from build123d import *

# Parameters (mm, degrees)
SKETCH1_R           = 11
SKETCH1_R_2         = 9.5
BOSS_EXTRUDE1_DEPTH = 10
BOSS_EXTRUDE2_START = -3
SKETCH2_R           = 11
SKETCH2_R_2         = 10
BOSS_EXTRUDE2_DEPTH = 3
SKETCH4_R           = 9.5
SKETCH4_R_2         = 8.5
BOSS_EXTRUDE3_DEPTH = 4


with BuildPart() as part:
    # Sketch1 → Boss-Extrude1 (new body)
    with BuildSketch(Plane.XY):
        with BuildLine():
            Line((-27.5, -15), (27.5, -15))
            ThreePointArc((27.5, -15), (42.5, 0), (27.5, 15))
            Line((27.5, 15), (9.069178574, 15))
            ThreePointArc((9.069178574, 15), (0, 18.5), (-9.069178574, 15))
            Line((-9.069178574, 15), (-27.5, 15))
            ThreePointArc((-27.5, 15), (-42.5, 0), (-27.5, -15))
        make_face()
        with Locations((-27.5, 0)):
            Circle(SKETCH1_R, mode=Mode.SUBTRACT)
        with Locations((27.5, 0)):
            Circle(SKETCH1_R, mode=Mode.SUBTRACT)
        with Locations((0, 5)):
            Circle(SKETCH1_R_2, mode=Mode.SUBTRACT)
    extrude(amount=BOSS_EXTRUDE1_DEPTH)

    # Sketch2 → Boss-Extrude2 (add)
    # profile 1 of 2: a face of its own
    with BuildSketch(Plane.XY.offset(10).offset(BOSS_EXTRUDE2_START)):
        with Locations((-27.5, 0)):
            Circle(SKETCH2_R)
        with Locations((-27.5, 0)):
            Circle(SKETCH2_R_2, mode=Mode.SUBTRACT)
    # profile 2 of 2: a face of its own
    with BuildSketch(Plane.XY.offset(10).offset(BOSS_EXTRUDE2_START)):
        with Locations((27.5, 0)):
            Circle(SKETCH2_R)
        with Locations((27.5, 0)):
            Circle(SKETCH2_R_2, mode=Mode.SUBTRACT)
    extrude(amount=BOSS_EXTRUDE2_DEPTH)

    # Sketch4 → Boss-Extrude3 (add)
    with BuildSketch(Plane(origin=(0, 0, 0), x_dir=(-1, 0, 0), z_dir=(0, 0, -1))):
        with Locations((0, 5)):
            Circle(SKETCH4_R)
        with Locations((0, 5)):
            Circle(SKETCH4_R_2, mode=Mode.SUBTRACT)
    extrude(amount=-BOSS_EXTRUDE3_DEPTH)


solid = part.part
Source: CAD feature listing. Evaluate the final solid. Frame: model axes, mm. A direction names the side the tool comes from. Round coordinates to 2 decimals unless told otherwise and drop trailing zeros. Loops run counter-clockwise (first coordinate to the right, second up) from the corner with the lowest first, then second, coordinate; pieces in that order, holes last.
Q1. Mould query, pull axis Y, two halves, no side actions, for faces 1 (the face through (-1, -5, 10)), 2 (the face through (37.661, -4.213, 3.451)), 3 (the face through (5.11, 13.01, 6.96)), 4 (the face through (-42.496, 0.33, 4.93)). Classes: pulls with the +Y half, pulls with the -Y half, needs draft (parallel to the pull), parting line crosses it, or undercut.
Q2. Section D-D, the plane y = 2. Return loops of the section in (x, z), plus the area to 3 significant figures.
Q3. First-contact query: P1, Ø10, axis at x = 0, y = 5, coming from the -Z side; P2, Ø5, axis at x = 14.5, z = 6, coming from the +Y side; P3, Ø1.5, axis at y = 7.5, z = 6.5, coming from the -X side; P4, Ø2, axis at y = 8, z = 8, coming from the +X side. Flat tips, straight axial feed; report the tip coordinate or a pass-through.
Q4. Section B-B, the plane z = 3.25. Return loops of the section in (x, y).
Q5. Section A-A, the plane x = 0. Return loops of the section in (y, z).
Q6. Section C-C, the plane y = 7.5. Return loops of the section in (x, z).
Q7. Ray query, line 1 (Y direction, x = -27.5, z = 7.7); line 2 (Y direction, x = 27, z = 3.5); line 3 (X direction, y = 3.5, z = 8). Return the intervals inside material, ascending.
Q8. Access query for faces 5 (the face through (2.2, -3.4, 4)), 6 (the face through (18, 15, 5)), 7 (the face through (-18, 15, 5)). Directions: +Z, -Z, +X, -X, +Y, -Y. A direction counts if a zero-diameter tool reaches every point of the face in a straight line with its end or side. Return the directions, or none.
Solutions:
1. face 1: needs draft
1. face 2: undercut
1. face 3: undercut
1. face 4: parting line crosses it
2. outline: (-42.37, 0) - (-38.32, 0) - (-38.32, 7) - (-37.3, 7) - (-37.3, 10) - (-42.37, 10) - close; (-17.7, 7) - (-16.68, 7) - (-16.68, 0) - (-7.95, 0) - (-7.95, 4) - (-9.01, 4) - (-9.01, 10) - (-17.7, 10) - close; (7.95, 0) - (16.68, 0) - (16.68, 7) - (17.7, 7) - (17.7, 10) - (9.01, 10) - (9.01, 4) - (7.95, 4) - close; (37.3, 7) - (38.32, 7) - (38.32, 0) - (42.37, 0) - (42.37, 10) - (37.3, 10) - close
2. area: 255 mm2
3. P1: passes through
3. P2: stops at y = 15
3. P3: stops at x = -40.9
3. P4: stops at x = 40.77
4. outline: (-27.5, -15) - (27.5, -15) arc R15 ccw to (27.5, 15) - (9.07, 15) arc R13.5 ccw to (-9.07, 15) - (-27.5, 15) arc R15 ccw to start; hole circle Ø22 at (-27.5, 0); hole circle Ø17 at (0, 5); hole circle Ø22 at (27.5, 0)
5. outline: (-15, 0) - (-3.5, 0) - (-3.5, 4) - (-4.5, 4) - (-4.5, 10) - (-15, 10) - close; (13.5, 0) - (18.5, 0) - (18.5, 10) - (14.5, 10) - (14.5, 4) - (13.5, 4) - close
6. outline: (-40.49, 0) - (-35.55, 0) - (-35.55, 7) - (-34.11, 7) - (-34.11, 10) - (-40.49, 10) - close; (-20.89, 7) - (-19.45, 7) - (-19.45, 0) - (-8.12, 0) - (-8.12, 4) - (-9.17, 4) - (-9.17, 10) - (-20.89, 10) - close; (8.12, 0) - (19.45, 0) - (19.45, 7) - (20.89, 7) - (20.89, 10) - (9.17, 10) - (9.17, 4) - (8.12, 4) - close; (34.11, 7) - (35.55, 7) - (35.55, 0) - (40.49, 0) - (40.49, 10) - (34.11, 10) - close
7. line 1: y = -15 to -10, 10 to 15
7. line 2: y = -15 to -10.99, 10.99 to 15
7. line 3: x = -42.09 to -36.87, -18.13 to -9.38, 9.38 to 18.13, 36.87 to 42.09
8. face 5: +Z
8. face 6: +Z, -Z, +X, +Y
8. face 7: +Z, -Z, -X, +Y
